```python
from build123d import *

# Parameters (mm, degrees)
RAIL_PROFILE_DEPTH             = 125
CBORE_FOR_M3_SHCS1_D           = 3.5
CBORE_FOR_M3_SHCS1_CBORE_D     = 6
CBORE_FOR_M3_SHCS1_CBORE_DEPTH = 4.5
FILL_START                     = -2.000000001
FILL_PATTERN1_OUTLINE_R        = 3
FILL_PATTERN1_DEPTH            = 4.5
FILL_START_2                   = -5.5
FILL_PATTERN1_2_OUTLINE_R      = 1.75
FILL_PATTERN1_2_DEPTH          = 3.499999999


# Read off the part's stored shape, not the designer's step: Fill Pattern1
with BuildPart() as part:
    # Sketch1 → RAIL PROFILE (new, symmetric)
    with BuildSketch(Plane.XY):
        with BuildLine():
            Line((-5.982334879, -1.370069213), (-5.982334879, -5.001472146))
            Line((-5.982334879, -5.001472146), (-5.483807025, -5.499999999))
            Line((-5.483807025, -5.499999999), (1.595289228, -5.499999999))
            ThreePointArc((1.595289228, -5.499999999), (1.994111552, -5.300588838), (2.392933875, -5.5))
            Line((2.392933875, -5.5), (5.483807024, -5.5))
            Line((5.483807024, -5.5), (5.982334878, -5.001472147))
            Line((5.982334878, -5.001472147), (5.982334878, -1.370069213))
            ThreePointArc((5.982334878, -1.370069213), (5.940056641, -1.231182813), (5.82756375, -1.139410101))
            ThreePointArc((5.82756375, -1.139410101), (5.497041405, -0.930122348), (5.251697363, -0.625405104))
            ThreePointArc((5.251697363, -0.625405104), (5.169975597, -0.541388466), (5.058890009, -0.504008866))
            Line((5.058890009, -0.504008866), (4.71429032, -0.473860299))
            ThreePointArc((4.71429032, -0.473860299), (4.552238438, -0.393945155), (4.486751147, -0.225544865))
            Line((4.486751147, -0.225544865), (4.486751147, 0.225544865))
            ThreePointArc((4.486751147, 0.225544865), (4.552238438, 0.393945155), (4.71429032, 0.473860299))
            Line((4.71429032, 0.473860299), (5.079776582, 0.505836204))
            ThreePointArc((5.079776582, 0.505836204), (5.187925163, 0.5413949), (5.268982803, 0.621333598))
            ThreePointArc((5.268982803, 0.621333598), (5.511607978, 0.899707672), (5.82756375, 1.09083865))
            ThreePointArc((5.82756375, 1.09083865), (5.940040963, 1.182638806), (5.982312115, 1.321532803))
            Line((5.982312115, 1.321532803), (5.982321902, 2.00145917))
            Line((5.982321902, 2.00145917), (5.483807025, 2.499999999))
            Line((5.483807025, 2.499999999), (-5.483807026, 2.499999999))
            Line((-5.483807026, 2.499999999), (-5.982321903, 2.00145917))
            Line((-5.982321903, 2.00145917), (-5.982321903, 1.32884687))
            ThreePointArc((-5.982321903, 1.32884687), (-5.942177076, 1.185718341), (-5.827697321, 1.090893402))
            ThreePointArc((-5.827697321, 1.090893402), (-5.511663234, 0.899754111), (-5.268982805, 0.621333597))
            ThreePointArc((-5.268982805, 0.621333597), (-5.187925164, 0.541394898), (-5.079776582, 0.505836204))
            Line((-5.079776582, 0.505836204), (-4.71429032, 0.473860299))
            ThreePointArc((-4.71429032, 0.473860299), (-4.552238438, 0.393945155), (-4.486751147, 0.225544865))
            Line((-4.486751147, 0.225544865), (-4.486751147, -0.225544865))
            ThreePointArc((-4.486751147, -0.225544865), (-4.552238438, -0.393945155), (-4.71429032, -0.473860299))
            Line((-4.71429032, -0.473860299), (-5.058890009, -0.504008866))
            ThreePointArc((-5.058890009, -0.504008866), (-5.169975597, -0.541388466), (-5.251697363, -0.625405104))
            ThreePointArc((-5.251697363, -0.625405104), (-5.499180752, -0.921502608), (-5.828043428, -1.123421157))
            ThreePointArc((-5.828043428, -1.123421157), (-5.944906256, -1.221900029), (-5.982334879, -1.370069213))
        make_face()
    extrude(amount=RAIL_PROFILE_DEPTH, both=True)

    # CBORE for M3 SHCS1 (through all)
    with Locations(Plane(origin=(0, 2.499999999, 0), x_dir=(1, 0, 0), z_dir=(0, 1, 0))):
        with Locations((0, 115)):
            cbore_for_m3_shcs1 = CounterBoreHole(CBORE_FOR_M3_SHCS1_D / 2, CBORE_FOR_M3_SHCS1_CBORE_D / 2, CBORE_FOR_M3_SHCS1_CBORE_DEPTH)

    # M3 END MIRROR: CBORE for M3 SHCS1 across plane
    add(cbore_for_m3_shcs1.mirror(Plane.XY), mode=Mode.SUBTRACT)

    # Fill Pattern1 outline → Fill Pattern1 (cut)
    with BuildSketch(Plane(origin=(0, 0, 0), x_dir=(1, 0, 0), z_dir=(0, 1, 0)).offset(FILL_START)):
        with Locations((0, 90)):
            Circle(FILL_PATTERN1_OUTLINE_R)
        with Locations((0, 65)):
            Circle(FILL_PATTERN1_OUTLINE_R)
        with Locations((0, 40)):
            Circle(FILL_PATTERN1_OUTLINE_R)
        with Locations((0, 15)):
            Circle(FILL_PATTERN1_OUTLINE_R)
        with Locations((0, -10)):
            Circle(FILL_PATTERN1_OUTLINE_R)
        with Locations((0, -35)):
            Circle(FILL_PATTERN1_OUTLINE_R)
        with Locations((0, -60)):
            Circle(FILL_PATTERN1_OUTLINE_R)
        with Locations((0, -85)):
            Circle(FILL_PATTERN1_OUTLINE_R)
    extrude(amount=FILL_PATTERN1_DEPTH, mode=Mode.SUBTRACT)

    # Fill Pattern1 2 outline → Fill Pattern1 2 (cut)
    with BuildSketch(Plane(origin=(0, 0, 0), x_dir=(1, 0, 0), z_dir=(0, 1, 0)).offset(FILL_START_2)):
        with Locations((0, 90)):
            Circle(FILL_PATTERN1_2_OUTLINE_R)
        with Locations((0, 65)):
            Circle(FILL_PATTERN1_2_OUTLINE_R)
        with Locations((0, 40)):
            Circle(FILL_PATTERN1_2_OUTLINE_R)
        with Locations((0, 15)):
            Circle(FILL_PATTERN1_2_OUTLINE_R)
        with Locations((0, -10)):
            Circle(FILL_PATTERN1_2_OUTLINE_R)
        with Locations((0, -35)):
            Circle(FILL_PATTERN1_2_OUTLINE_R)
        with Locations((0, -60)):
            Circle(FILL_PATTERN1_2_OUTLINE_R)
        with Locations((0, -85)):
            Circle(FILL_PATTERN1_2_OUTLINE_R)
    extrude(amount=FILL_PATTERN1_2_DEPTH, mode=Mode.SUBTRACT)


solid = part.part
```
Model file for the job. Use its own axes, mm. A direction names the side the tool comes from. Coordinates: 2 decimals unless noted, no trailing zeros. Return JSON: item names as keys, results as strings. Group by question number.
1) Probe line 1 (Y direction, x = 5, z = 15.5); line 2 (X direction, y = 0.1, z = 85); line 3 (X direction, y = -3, z = -115). List the from-to ranges inside material, lowest first. Write a range as from..to.
2) Tool access for faces 1 (the flat face through (-2, -5.5, 2)), 2 (the cylindrical face through (0, 0, 7)): list every direction of +Z, -Z, +X, -X, +Y, -Y with a clear straight run to the whole face (end or side of a thin tool).
3) Flat gauge pins, fed straight in: P1, Ø5.5, axis at x = 0, z = -115, coming from the +Y side; P2, Ø0.5, axis at y = 0, z = -6, coming from the +X side. Where does each tip first touch, or does it go through?
4) Mould opens along X. For faces 3 (the cylindrical face through (0, 0, 57)), 4 (the flat face through (0, -1, -125)) say: released by +X, released by -X, zero draft, split by the parting line, or undercut.
Values found:
{
 "1": {"line 1": "y = -5.5..-0.5, 0.5..2.5", "line 2": "x = -4.49..-3, 3..4.49", "line 3": "x = -5.98..-1.75, 1.75..5.98"},
 "2": {"face 1": "+Z, -Z, +X, -X, -Y", "face 2": "+Y"},
 "3": {"P1": "stops at y = -2", "P2": "stops at x = 4.49"},
 "4": {"face 3": "undercut", "face 4": "zero draft"}
}
